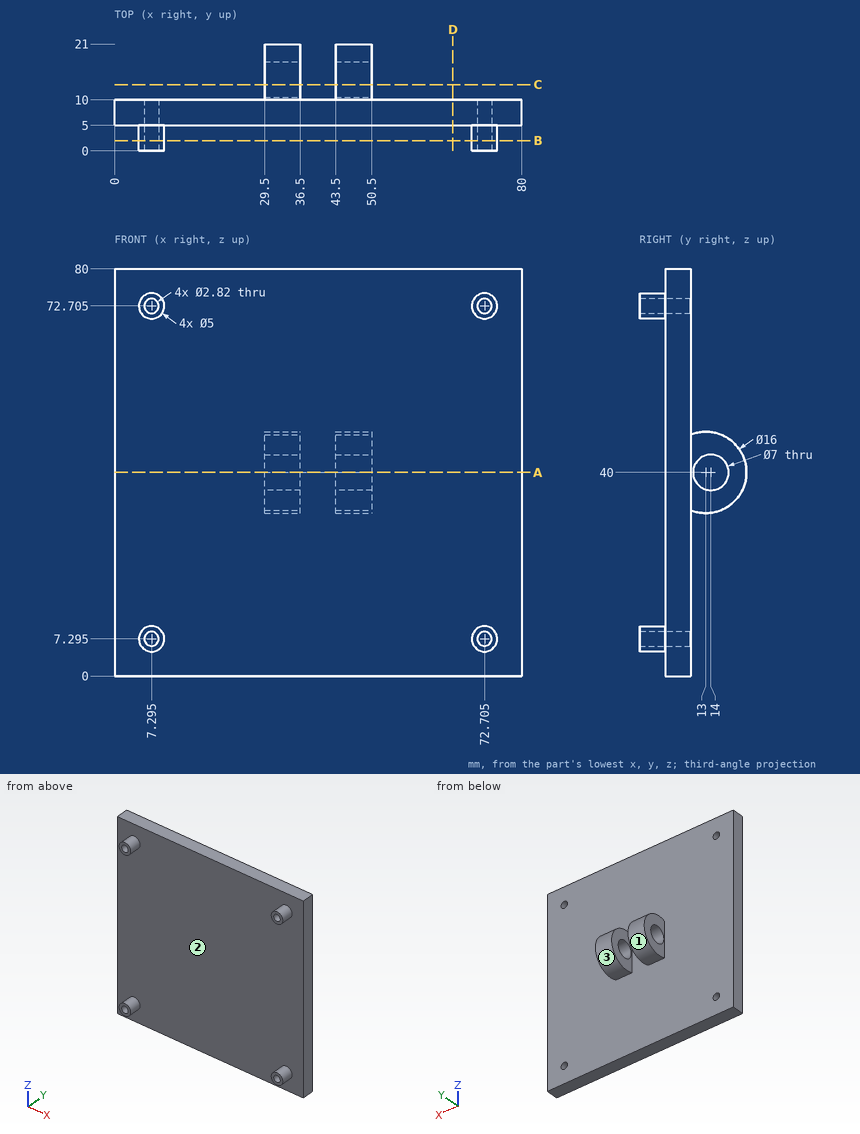
Geometry check sheet. Reference: drawing and pictorial views, mm from the part's lowest x, y, z. Round coordinates to 2 decimals unless told otherwise and drop trailing zeros. Write each loop counter-clockwise with the first axis right and the second up, starting at its lowest first coordinate (ties: lowest second). Pieces come first, ordered by that corner, then holes. Notation, with made-up numbers: (16, 23.25) -> (46, 23.25) arc R18 cw to (46, 40.25) -> close; hole circle Ø4 at (-0.75, 37). An arc over 180 degrees is marked (long way). Put each result on its own line as item: value.
1) Depth check by flat-ended pin: P1, Ø2, axis at x = 13, z = 32.5, coming from the -Y side; P2, Ø4.5, axis at x = 72.705, z = 7.295, coming from the +Y side; P3, Ø3.5, axis at y = 15, z = 36.5, coming from the -X side. Enter the tip coordinate at first touch or a pass-through.
Recorded:
P1: stops at y = 5
P2: stops at y = 10
P3: stops at x = 29.5
2) Cross-section at C-C, the plane y = 13. Enter the section's corners in (x, z).
Recorded:
outline: (29.5, 32) -> (36.5, 32) -> (36.5, 36.65) -> (29.5, 36.65) -> close; (29.5, 43.35) -> (36.5, 43.35) -> (36.5, 48) -> (29.5, 48) -> close; (43.5, 32) -> (50.5, 32) -> (50.5, 36.65) -> (43.5, 36.65) -> close; (43.5, 43.35) -> (50.5, 43.35) -> (50.5, 48) -> (43.5, 48) -> close
3) Thickness scan on probe 1 along Z at (x, y) = (7.5, 3.5); probe 2 along X at (y, z) = (18.75, 38); probe 3 along Y at (x, z) = (67.5, 52.5). Record the ranges inside material, lowest first. Write a range as from..to.
Recorded:
probe 1: z = 4.8..5.9, 8.69..9.79, 70.21..71.31, 74.1..75.2
probe 2: x = 29.5..36.5, 43.5..50.5
probe 3: y = 5..10
4) Cross-section at A-A, the plane z = 40. Enter the section's corners in (x, y), plus the area to 3 significant figures.
Recorded:
outline: (0, 5) -> (80, 5) -> (80, 10) -> (50.5, 10) -> (50.5, 10.5) -> (43.5, 10.5) -> (43.5, 10) -> (36.5, 10) -> (36.5, 10.5) -> (29.5, 10.5) -> (29.5, 10) -> (0, 10) -> close; (29.5, 17.5) -> (36.5, 17.5) -> (36.5, 21) -> (29.5, 21) -> close; (43.5, 17.5) -> (50.5, 17.5) -> (50.5, 21) -> (43.5, 21) -> close
area: 456 mm2
5) Cross-section at B-B, the plane y = 2. Enter the section's corners in (x, z) (3 decimals), plus the area to 3 significant figures.
Recorded:
outline: circle Ø5 at (7.295, 7.295); circle Ø5 at (7.295, 72.705); circle Ø5 at (72.705, 7.295); circle Ø5 at (72.705, 72.705); hole circle Ø2.82 at (7.295, 7.295); hole circle Ø2.82 at (7.295, 72.705); hole circle Ø2.82 at (72.705, 7.295); hole circle Ø2.82 at (72.705, 72.705)
area: 53.6 mm2
6) Release check for a two-part mould opening along Y. For the marked faces 1, 2 and 3 record: pulls with the +Y half, pulls with the -Y half, needs draft (parallel to the pull), parting line crosses it, or undercut.
Recorded:
face 1: undercut
face 2: pulls with the -Y half
face 3: undercut
7) Cross-section at D-D, the plane x = 66.5. Enter the section's corners in (y, z), plus the area to 3 significant figures.
Recorded:
outline: (5, 0) -> (10, 0) -> (10, 80) -> (5, 80) -> close
area: 400 mm2
